Read the model definition and answer for the solid it produces. Units are mm, in the model's axes. A direction names the side the tool comes from. Coordinates: 2 decimals unless noted, no trailing zeros. Write each loop counter-clockwise with the first axis right and the second up, starting at its lowest first coordinate (ties: lowest second). Pieces come first, ordered by that corner, then holes. Notation, with made-up numbers: (18, 0.5) - (58, 0.5) arc R18 cw to (58, 14.5) - close; hole circle Ø8 at (56, 62.25). An arc over 180 degrees is marked (long way). Use a Markdown table: item, result.
from build123d import *

# Parameters (mm, degrees)
F0_R     = 18.5
F1_DEPTH = 52
F2_SIZE2 = 1.5
F2_SIZE  = 5
F3_R     = 47
F4_DEPTH = 5.5
F6_R     = 7.9375
F7_DEPTH = 57.501


# Not quite as in the source:
# - a fillet or chamfer that OpenCascade refuses, or shapes differently, is made with other operations: its cross-section is extruded or revolved along the edge and cut away or added


with BuildPart() as f1:
    # F0 (on Top) → F1 (new body)
    with BuildSketch(Plane.XY):
        Circle(F0_R)
    extrude(amount=F1_DEPTH)

    # F2
    f2_edges = [f1.edges().sort_by_distance(p)[0] for p in [
        (-18.5, 0, 0),
    ]]
    f2_side = f1.faces().sort_by_distance((-18.5, 0, 26))[0]
    chamfer(f2_edges, length=F2_SIZE, length2=F2_SIZE2, reference=f2_side)

    # F3 (on face) → F4 (join)
    with BuildSketch(Plane.XY.offset(52)):
        Circle(F3_R)
    extrude(amount=F4_DEPTH)

    # F5: chamfer of 1 x 10.2 on 1 edges, made by hand

    # F5_s1 → F5_t2 (revolve, cut)
    with BuildSketch(Plane.XZ):
        Polygon((47, 47.3), (46, 57.5), (47, 57.5), align=None)
    revolve(axis=Axis((0, 0, 57.5), (0, 0, 1)), mode=Mode.SUBTRACT)

    # F6 (on face) → F7 (cut, through all)
    with BuildSketch(Plane.XY.offset(57.5)):
        Circle(F6_R)
    extrude(amount=-F7_DEPTH, mode=Mode.SUBTRACT)


solid = f1.part
(1) A cutting plane is placed at A-A, the plane x = 0. Write down the section's boundary in (y, z).
Report:
| item | result |
|---|---|
| outline | (-46.54, 52) - (-18.5, 52) - (-18.5, 5) - (-17, 0) - (-7.94, 0) - (-7.94, 57.5) - (-46, 57.5) - close; (7.94, 0) - (17, 0) - (18.5, 5) - (18.5, 52) - (46.54, 52) - (46, 57.5) - (7.94, 57.5) - close |
(2) For faces 1 (the cylindrical face through (-4.01, -18.06, 28.17)), 2 (the flat face through (7.3, -3.5, 0)), determine the directions among +Z, -Z, +X, -X, +Y, -Y from which every point of the face is accessible in a straight line to the end or side of a thin tool.
Report:
| item | result |
|---|---|
| face 1 | -Z |
| face 2 | -Z, +X, -X, +Y, -Y |
(3) Each of these flat-tipped pins is pushed along its axis until it touches: P1, Ø12.5, axis at x = 0, y = 0, coming from the -Z side; P2, Ø5, axis at y = 17, z = 30, coming from the -X side; P3, Ø1, axis at x = 37, y = -10, coming from the -Z side; P4, Ø3, axis at y = -9.5, z = 12.5, coming from the +X side. Where does it stop, or does it pass through?
Report:
| item | result |
|---|---|
| P1 | passes through |
| P2 | stops at x = -11.49 |
| P3 | stops at z = 52 |
| P4 | stops at x = 16.68 |
(4) Straight lines are drawn through the part: L1, parallel to Y at x = 0, z = 40; L2, parallel to Z at x = 21, y = 38.5; L3, parallel to X at y = -4, z = 50.5. For each, find the intervals that lie inside material, in ascending order.
Report:
| item | result |
|---|---|
| L1 | y = -18.5 to -7.94, 7.94 to 18.5 |
| L2 | z = 52 to 57.5 |
| L3 | x = -18.06 to -6.86, 6.86 to 18.06 |
(5) A cutting plane is placed at C-C, the plane z = 30.5. Write down the section's boundary in (x, y) (1 decimal), and give its area (3 significant figures).
Report:
| item | result |
|---|---|
| outline | circle Ø37 at (0, 0); hole circle Ø15.9 at (0, 0) |
| area | 877 mm² |
(6) The mould has two halves that part along Y. Classify faces 3 (the cylindrical face through (-1.72, -7.75, 29.15)), 4 (the conical face through (21.238, -40.833, 57.233)), 5 (the flat face through (20, 1, 52)): pulls with the +Y half, pulls with the -Y half, needs draft (parallel to the pull), parting line crosses it, or undercut.
Report:
| item | result |
|---|---|
| face 3 | undercut |
| face 4 | parting line crosses it |
| face 5 | needs draft |
